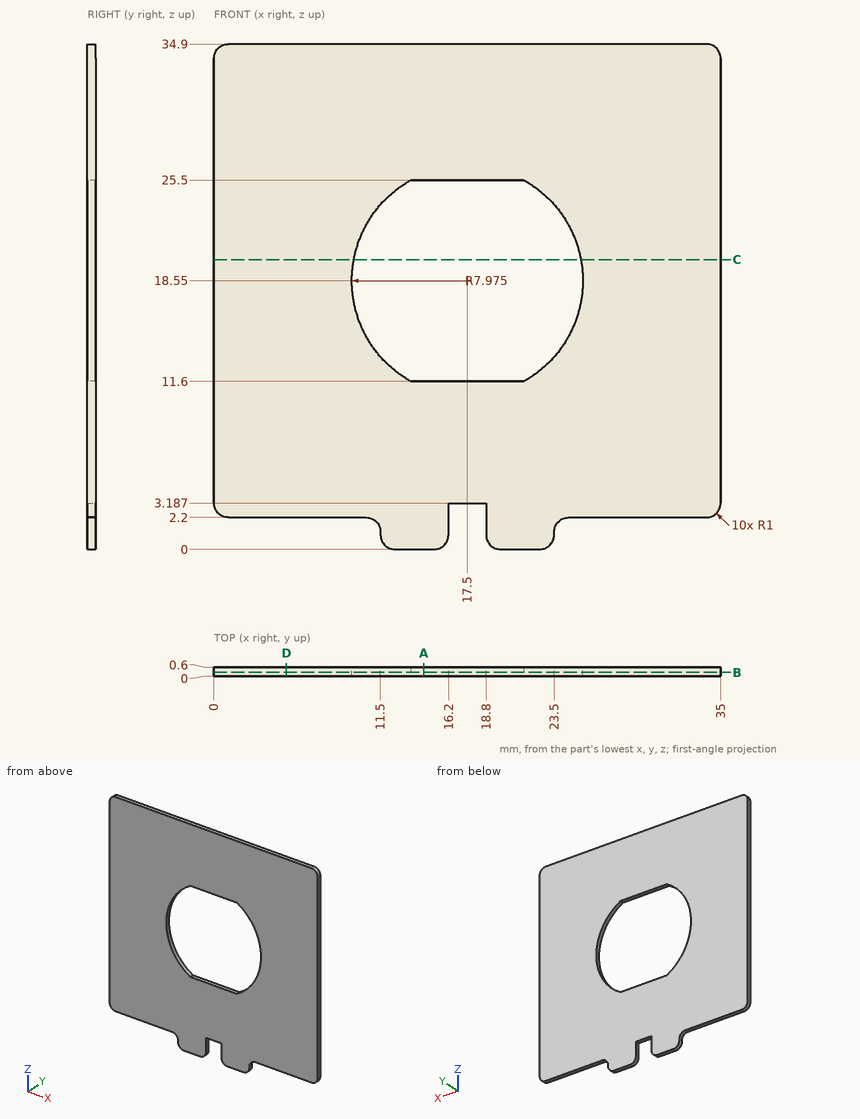
Verification items for this drawing (mm, ordinates from the low corner). Give positions to 0.01 mm unless a question says otherwise; leave off trailing zeros. Write each loop counter-clockwise with the first axis right and the second up, starting at its lowest first coordinate (ties: lowest second). Pieces come first, ordered by that corner, then holes. Notation, with made-up numbers: (75, -39.5) -> (134, -39.5) arc R20 cw to (134, -34.5) -> close; hole circle Ø11 at (43.5, 53.5). An arc over 180 degrees is marked (long way). Use CSV: the item, a comma, the result in double quotes. Start each with the question number.
Q1. Cross-section at B-B on y = 0.25. Enter the section's corners in (x, z) (3 decimals).
Q2. Scan lines: line 1 along Z through (x, y) = (19, 0.55); line 2 along Z through (x, y) = (26, 0.35); line 3 along X through (y, z) = (0.15, 19.5). Record each from-to range of solid material in increasing order.
Q3. Cross-section at A-A on x = 14.5. Enter the section's corners in (y, z), and give its area (3 significant figures).
Q4. Cross-section at C-C on z = 20. Enter the section's corners in (x, y), and give its area (3 significant figures).
Q5. Cross-section at D-D on x = 5. Enter the section's corners in (y, z), and give its area (3 significant figures).
Working result:
1,outline,"(0, 3.2) arc R1 ccw to (1, 2.2) -> (10.5, 2.2) arc R1 cw to (11.5, 1.2) -> (11.5, 1) arc R1 ccw to (12.5, 0) -> (15.2, 0) arc R1 ccw to (16.2, 1) -> (16.2, 3.187) -> (18.8, 3.187) -> (18.8, 1) arc R1 ccw to (19.8, 0) -> (22.5, 0) arc R1 ccw to (23.5, 1) -> (23.5, 1.2) arc R1 cw to (24.5, 2.2) -> (34, 2.2) arc R1 ccw to (35, 3.2) -> (35, 33.9) arc R1 ccw to (34, 34.9) -> (1, 34.9) arc R1 ccw to (0, 33.9) -> close; hole (13.589, 11.6) -> (21.411, 11.6) arc R7.975 ccw to (21.411, 25.5) -> (13.589, 25.5) arc R7.975 ccw to start"
2,line 1,"z = 0.4 to 11.6, 25.5 to 34.9"
2,line 2,"z = 2.2 to 34.9"
2,line 3,"x = 0 to 9.58, 25.42 to 35"
3,outline,"(0, 0) -> (0.6, 0) -> (0.6, 11.6) -> (0, 11.6) -> close; (0, 25.5) -> (0.6, 25.5) -> (0.6, 34.9) -> (0, 34.9) -> close"
3,area,"12.6 mm^2"
4,outline,"(0, 0) -> (9.66, 0) -> (9.66, 0.6) -> (0, 0.6) -> close; (25.34, 0) -> (35, 0) -> (35, 0.6) -> (25.34, 0.6) -> close"
4,area,"11.6 mm^2"
5,outline,"(0, 2.2) -> (0.6, 2.2) -> (0.6, 34.9) -> (0, 34.9) -> close"
5,area,"19.6 mm^2"
